Could you check a few things on this model? Use its own coordinates, in mm. Face numbers are marked on the shaded views. Round coordinates to 2 decimals unless told otherwise and drop trailing zeros. Loops run counter-clockwise (first coordinate to the right, second up) from the corner with the lowest first, then second, coordinate; pieces in that order, holes last. Notation, with made-up numbers: M 6,29.25 L 58,29.25 A19 cw 58,47.25 Z; hole C 6.5,-36.75 d6. An arc over 180 degrees is marked long. Answer in a Markdown table with one row per item.
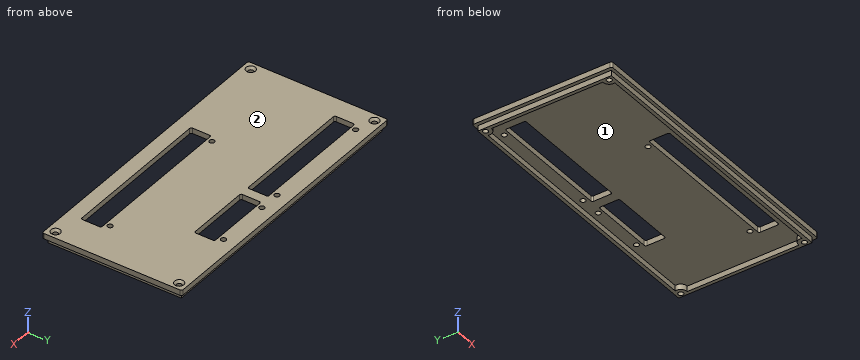
```python
from build123d import *

# Parameters (mm, degrees)
F0_R           = 1.1938
F1_DEPTH       = 2.54
F2_W           = 132.4737
F2_H           = 62.23
F3_DEPTH       = 2.54
F4_D           = 2.3876
F4_CSINK_D     = 4.318
F4_CSINK_ANGLE = 82


with BuildPart() as f1:
    # F0 (on Top) → F1 (new body)
    with BuildSketch(Plane.XY):
        with BuildLine():
            ThreePointArc((-763.551821, 381.242233), (-763.784305, 381.803499), (-764.345571, 382.035983))
            Line((-764.345571, 382.035983), (-898.635371, 382.035983))
            ThreePointArc((-898.635371, 382.035983), (-899.196637, 381.803499), (-899.429121, 381.242233))
            Line((-899.429121, 381.242233), (-899.429121, 317.729533))
            ThreePointArc((-899.429121, 317.729533), (-899.196637, 317.168267), (-898.635371, 316.935783))
            Line((-898.635371, 316.935783), (-764.345571, 316.935783))
            ThreePointArc((-764.345571, 316.935783), (-763.784305, 317.168267), (-763.551821, 317.729533))
            Line((-763.551821, 317.729533), (-763.551821, 381.242233))
        make_face()
        with Locations((-849.200621, 335.528583)):
            Circle(F0_R, mode=Mode.SUBTRACT)
        with BuildLine():
            ThreePointArc((-780.118971, 333.293383), (-779.557705, 333.060899), (-779.325221, 332.499633))
            Line((-779.325221, 332.499633), (-779.325221, 324.574833))
            ThreePointArc((-779.325221, 324.574833), (-779.557705, 324.013567), (-780.118971, 323.781083))
            Line((-780.118971, 323.781083), (-851.124671, 323.781083))
            ThreePointArc((-851.124671, 323.781083), (-851.685937, 324.013567), (-851.918421, 324.574833))
            Line((-851.918421, 324.574833), (-851.918421, 332.499633))
            ThreePointArc((-851.918421, 332.499633), (-851.685937, 333.060899), (-851.124671, 333.293383))
            Line((-851.124671, 333.293383), (-780.118971, 333.293383))
        make_face(mode=Mode.SUBTRACT)
        with Locations((-782.043021, 335.528583)):
            Circle(F0_R, mode=Mode.SUBTRACT)
        with Locations((-886.970421, 375.863783)):
            Circle(F0_R, mode=Mode.SUBTRACT)
        with BuildLine():
            Line((-888.894471, 373.603183), (-833.128771, 373.603183))
            ThreePointArc((-833.128771, 373.603183), (-832.567505, 373.370699), (-832.335021, 372.809433))
            Line((-832.335021, 372.809433), (-832.335021, 364.884633))
            ThreePointArc((-832.335021, 364.884633), (-832.567505, 364.323367), (-833.128771, 364.090883))
            Line((-833.128771, 364.090883), (-888.894471, 364.090883))
            ThreePointArc((-888.894471, 364.090883), (-889.455737, 364.323367), (-889.688221, 364.884633))
            Line((-889.688221, 364.884633), (-889.688221, 372.809433))
            ThreePointArc((-889.688221, 372.809433), (-889.455737, 373.370699), (-888.894471, 373.603183))
        make_face(mode=Mode.SUBTRACT)
        with Locations((-835.052821, 375.863783)):
            Circle(F0_R, mode=Mode.SUBTRACT)
        with BuildLine():
            Line((-826.994671, 373.603183), (-797.898971, 373.603183))
            ThreePointArc((-797.898971, 373.603183), (-797.337705, 373.370699), (-797.105221, 372.809433))
            Line((-797.105221, 372.809433), (-797.105221, 364.884633))
            ThreePointArc((-797.105221, 364.884633), (-797.337705, 364.323367), (-797.898971, 364.090883))
            Line((-797.898971, 364.090883), (-826.994671, 364.090883))
            ThreePointArc((-826.994671, 364.090883), (-827.555937, 364.323367), (-827.788421, 364.884633))
            Line((-827.788421, 364.884633), (-827.788421, 372.809433))
            ThreePointArc((-827.788421, 372.809433), (-827.555937, 373.370699), (-826.994671, 373.603183))
        make_face(mode=Mode.SUBTRACT)
        with Locations((-825.070621, 375.863783)):
            Circle(F0_R, mode=Mode.SUBTRACT)
        with Locations((-799.823021, 375.863783)):
            Circle(F0_R, mode=Mode.SUBTRACT)
    extrude(amount=-F1_DEPTH)

    # F2 (on face) → F3 (join)
    with BuildSketch(Plane(origin=(0, 0, -2.54), x_dir=(1, 0, 0), z_dir=(0, 0, -1))):
        with Locations((-831.490471, -349.485883)):
            Rectangle(F2_W, F2_H)
        with BuildLine():
            ThreePointArc((-769.793631, -319.958383), (-769.219127, -322.459981), (-766.841121, -323.425971))
            Line((-766.841121, -323.425971), (-766.841121, -375.545795))
            ThreePointArc((-766.841121, -375.545795), (-769.219127, -376.511785), (-769.793631, -379.013383))
            Line((-769.793631, -379.013383), (-893.187311, -379.013383))
            ThreePointArc((-893.187311, -379.013383), (-893.761815, -376.511785), (-896.139821, -375.545795))
            Line((-896.139821, -375.545795), (-896.139821, -323.425971))
            ThreePointArc((-896.139821, -323.425971), (-893.761815, -322.459981), (-893.187311, -319.958383))
            Line((-893.187311, -319.958383), (-769.793631, -319.958383))
        make_face(mode=Mode.SUBTRACT)
    extrude(amount=F3_DEPTH)

    # F4 (through all)
    with Locations(Plane.XY):
        with Locations((-895.879471, 378.314883), (-767.101471, 378.314883), (-767.101471, 320.656883), (-895.879471, 320.656883)):
            CounterSinkHole(F4_D / 2, F4_CSINK_D / 2, counter_sink_angle=F4_CSINK_ANGLE)


solid = f1.part
```
1) I need wall thicknesses on line 1 (Y direction, x = -801.5, z = -1.3); line 2 (X direction, y = 327, z = -2.2); line 3 (Y direction, x = -860.5, z = -1.65). Which ranges of each line are inside material? Lowest first, please.
Computed:
| item | result |
|---|---|
| line 1 | y = 316.94 to 323.78, 333.29 to 364.09, 373.6 to 382.04 |
| line 2 | x = -899.43 to -851.92, -779.33 to -763.55 |
| line 3 | y = 316.94 to 364.09, 373.6 to 382.04 |
2) I want a section at B-B, the plane x = -867. Please give me the cut outline in (y, z), plus the area to 3 significant figures.
Computed:
| item | result |
|---|---|
| outline | M 316.94,-2.54 L 318.37,-2.54 L 318.37,-5.08 L 319.96,-5.08 L 319.96,-2.54 L 364.09,-2.54 L 364.09,0 L 316.94,0 Z; M 373.6,-2.54 L 379.01,-2.54 L 379.01,-5.08 L 380.6,-5.08 L 380.6,-2.54 L 382.04,-2.54 L 382.04,0 L 373.6,0 Z |
| area | 149 mm² |
3) I want a section at D-D, the plane y = 342.5. Please give me the cut outline in (x, z).
Computed:
| item | result |
|---|---|
| outline | M -899.43,-2.54 L -897.73,-2.54 L -897.73,-5.08 L -896.14,-5.08 L -896.14,-2.54 L -766.84,-2.54 L -766.84,-5.08 L -765.25,-5.08 L -765.25,-2.54 L -763.55,-2.54 L -763.55,0 L -899.43,0 Z |
4) If we mould it in two halves opening along Y, with no side actions, what happens to the marked faces 1 and 2? For each: released by +Y, released by -Y, zero draft, split by the parting line, or undercut.
Computed:
| item | result |
|---|---|
| face 1 | undercut |
| face 2 | zero draft |
5) I want a section at A-A, the plane x = -838.5. Please give me the cut outline in (y, z), plus the area to 3 significant figures.
Computed:
| item | result |
|---|---|
| outline | M 316.94,-2.54 L 318.37,-2.54 L 318.37,-5.08 L 319.96,-5.08 L 319.96,-2.54 L 323.78,-2.54 L 323.78,0 L 316.94,0 Z; M 333.29,-2.54 L 364.09,-2.54 L 364.09,0 L 333.29,0 Z; M 373.6,-2.54 L 379.01,-2.54 L 379.01,-5.08 L 380.6,-5.08 L 380.6,-2.54 L 382.04,-2.54 L 382.04,0 L 373.6,0 Z |
| area | 125 mm² |
6) Will these pins go through, and if not, where does the flat tip stop? P1, Ø2, axis at y = 369.5, z = -4.5, coming from the -X side; P2, Ø2, axis at x = -831.5, z = -4.5, coming from the -Y side; P3, Ø0.8, axis at y = 357, z = -4.5, coming from the +X side.
Computed:
| item | result |
|---|---|
| P1 | stops at x = -897.73 |
| P2 | stops at y = 318.37 |
| P3 | stops at x = -765.25 |
7) I want a section at C-C, the plane y = 327.5. Please give me the cut outline in (x, z).
Computed:
| item | result |
|---|---|
| outline | M -899.43,-2.54 L -897.73,-2.54 L -897.73,-5.08 L -896.14,-5.08 L -896.14,-2.54 L -851.92,-2.54 L -851.92,0 L -899.43,0 Z; M -779.33,-2.54 L -766.84,-2.54 L -766.84,-5.08 L -765.25,-5.08 L -765.25,-2.54 L -763.55,-2.54 L -763.55,0 L -779.33,0 Z |
